Geometry: final body of the model. Coordinates: model frame, mm. Round coordinates to 2 decimals unless told otherwise and drop trailing zeros. Order: outer loops, then holes, each group sorted by start corner. A loop starts at its lowest first (then second) coordinate and runs counter-clockwise, first axis right, second up. Notation, with made-up numbers: M -24.75,51 L 25.25,51 A9 cw 25.25,55 Z; hole C 33,40.25 d4. An arc over 180 degrees is marked long. Put each result on its own line as item: value. Start each with the question number.
1) Section B-B, the plane x = -14. Return loops of the section in (y, z).
2) Section A-A, the plane y = -1.25. Return loops of the section in (x, z), then the cut area to 3 significant figures.
3) First-contact query: P1, Ø1, axis at y = -0.5, z = 2, coming from the -X side. Flat tip, straight axial feed; report the tip coordinate or a pass-through.
4) Material intervals for probe 1 along X at (y, z) = (1, 1.9); probe 2 along X at (y, z) = (0.75, 2.15); probe 3 along Y at (x, z) = (-11.5, 2.3), sorted ascending. Write a range as [from, to].
from build123d import *

# Parameters (mm, degrees)
EXTRUDE_1_DEPTH = 3


with BuildPart() as part:
    # Эскиз1 → Бобышка-Вытянуть1 (new body)
    with BuildSketch(Plane.XY):
        with BuildLine():
            ThreePointArc((-6.6, 0), (-7.961953467, -3.288046533), (-11.25, -4.65))
            Line((-11.25, -4.65), (11.25, -4.65))
            ThreePointArc((11.25, -4.65), (6.6, 0), (11.25, 4.65))
            Line((11.25, 4.65), (-11.25, 4.65))
            ThreePointArc((-11.25, 4.65), (-7.961953467, 3.288046533), (-6.6, 0))
        make_face()
        with BuildLine():
            ThreePointArc((11.25, 4.65), (6.6, 0), (11.25, -4.65))
            Line((11.25, -4.65), (11.25, -1.65))
            ThreePointArc((11.25, -1.65), (9.6, 0), (11.25, 1.65))
            Line((11.25, 1.65), (11.25, 4.65))
        make_face()
        with BuildLine():
            Line((11.25, -1.65), (11.25, -4.65))
            ThreePointArc((11.25, -4.65), (14.538046533, -3.288046533), (15.9, 0))
            ThreePointArc((15.9, 0), (14.538046533, 3.288046533), (11.25, 4.65))
            Line((11.25, 4.65), (11.25, 1.65))
            ThreePointArc((11.25, 1.65), (12.416726189, 1.166726189), (12.9, 0))
            ThreePointArc((12.9, 0), (12.416726189, -1.166726189), (11.25, -1.65))
        make_face()
        with BuildLine():
            ThreePointArc((-11.25, 4.65), (-15.9, 0), (-11.25, -4.65))
            Line((-11.25, -4.65), (-11.25, -1.65))
            ThreePointArc((-11.25, -1.65), (-12.9, 0), (-11.25, 1.65))
            Line((-11.25, 1.65), (-11.25, 4.65))
        make_face()
        with BuildLine():
            Line((-11.25, -1.65), (-11.25, -4.65))
            ThreePointArc((-11.25, -4.65), (-7.961953467, -3.288046533), (-6.6, 0))
            ThreePointArc((-6.6, 0), (-7.961953467, 3.288046533), (-11.25, 4.65))
            Line((-11.25, 4.65), (-11.25, 1.65))
            ThreePointArc((-11.25, 1.65), (-10.083273811, 1.166726189), (-9.6, 0))
            ThreePointArc((-9.6, 0), (-10.083273811, -1.166726189), (-11.25, -1.65))
        make_face()
    extrude(amount=EXTRUDE_1_DEPTH)


solid = part.part
Result sheet:
1. outline: M -3.75,0 L 3.75,0 L 3.75,3 L -3.75,3 Z
2. outline: M -15.73,0 L -12.33,0 L -12.33,3 L -15.73,3 Z; M -10.17,0 L 10.17,0 L 10.17,3 L -10.17,3 Z; M 12.33,0 L 15.73,0 L 15.73,3 L 12.33,3 Z
2. area: 81.4 mm2
3. P1: stops at x = -15.9
4. probe 1: x = [-15.79, -12.56], [-9.94, 9.94], [12.56, 15.79]
4. probe 2: x = [-15.84, -12.72], [-9.78, 9.78], [12.72, 15.84]
4. probe 3: y = [-4.64, -1.63], [1.63, 4.64]
